from build123d import *

# Parameters (mm, degrees)
SKETCH1_R           = 1.5875
BOSS_EXTRUDE1_DEPTH = 6
CUT_EXTRUDE1_START  = 9
CUT_EXTRUDE1_DEPTH  = 2.1


with BuildPart() as part:
    # Sketch1 → Boss-Extrude1 (new body)
    with BuildSketch(Plane.XY):
        with BuildLine():
            Line((-9.16515139, -4), (-1.658312395, -2.5))
            ThreePointArc((-1.658312395, -2.5), (0, -3), (1.658312395, -2.5))
            Line((1.658312395, -2.5), (9.16515139, -4))
            ThreePointArc((9.16515139, -4), (10, 0), (9.16515139, 4))
            Line((9.16515139, 4), (1.658312395, 2.5))
            ThreePointArc((1.658312395, 2.5), (0, 3), (-1.658312395, 2.5))
            Line((-1.658312395, 2.5), (-9.16515139, 4))
            ThreePointArc((-9.16515139, 4), (-10, 0), (-9.16515139, -4))
        make_face()
        Circle(SKETCH1_R, mode=Mode.SUBTRACT)
    extrude(amount=BOSS_EXTRUDE1_DEPTH)

    # Sketch2 → Cut-Extrude1 (cut)
    with BuildSketch(Plane(origin=(0, 0, 0), x_dir=(0, 0, -1), z_dir=(1, 0, 0)).offset(CUT_EXTRUDE1_START)):
        with BuildLine():
            Line((-3, 2.1), (-5.1, 2.1))
            Line((-5.1, 2.1), (-5.1, -2.1))
            Line((-5.1, -2.1), (-3, -2.1))
            ThreePointArc((-3, -2.1), (-0.9, 0), (-3, 2.1))
        make_face()
    cut_extrude1 = extrude(amount=-CUT_EXTRUDE1_DEPTH, mode=Mode.SUBTRACT)

    # Mirror1: Cut-Extrude1 across plane
    add(cut_extrude1.mirror(Plane(origin=(0, 0, 0), x_dir=(0, 0, 1), z_dir=(1, 0, 0))), mode=Mode.SUBTRACT)


solid = part.part
The listing builds one solid part. Answer for the finished solid, in the listing's coordinates (mm). A direction names the side the tool comes from. Coordinates: 2 decimals unless noted, no trailing zeros. Order: outer loops, then holes, each group sorted by start corner. A loop starts at its lowest first (then second) coordinate and runs counter-clockwise, first axis right, second up. Notation, with made-up numbers: M 10.25,25 L 32.25,25 A10 cw 32.25,42 Z; hole C 14,-6.75 d5. An arc over 180 degrees is marked long. Use CSV: the item, a comma, the result in double quotes.
Q1. A tool of negligible diameter and unlimited length cuts with its end or side. For faces 4 (the flat face through (5.36, -3.24, 2.96)), 5 (the flat face through (0, -2, 0)), 6 (the flat face through (5.46, 3.26, 2.96)), 7 (the cylindrical face through (-0.34, -1.55, 2.96)), 8 (the flat face through (-6.9, 0, 3)), from which of +Z, -Z, +X, -X, +Y, -Y can it reach the whole face along a straight path? Write none if from no direction.
Here are the results:
face 4,"+Z, -Z, -Y"
face 5,"-Z, +X, -X, +Y, -Y"
face 6,"+Z, -Z, +Y"
face 7,"+Z, -Z"
face 8,"none"
Q2. Section B-B (z = 0.7) is taken. Determine the outline of the cut face in (x, y) (1 decimal).
Here are the results:
outline,"M -9.2,-4 L -1.7,-2.5 A3 ccw 1.7,-2.5 L 9.2,-4 A10 ccw 9.2,4 L 1.7,2.5 A3 ccw -1.7,2.5 L -9.2,4 A10 ccw Z; hole C 0,0 d3.2"
Q3. Section C-C (x = 0) is taken. Determine the outline of the cut face in (y, z).
Here are the results:
outline,"M -3,0 L -1.59,0 L -1.59,6 L -3,6 Z; M 1.59,0 L 3,0 L 3,6 L 1.59,6 Z"
Q4. Section A-A (y = 0) is taken. Determine the outline of the cut face in (x, z).
Here are the results:
outline,"M -10,0 L -1.59,0 L -1.59,6 L -10,6 Z; M 1.59,0 L 10,0 L 10,6 L 1.59,6 Z; hole M -9,0.9 L -6.9,0.9 L -6.9,5.1 L -9,5.1 Z; hole M 6.9,0.9 L 9,0.9 L 9,5.1 L 6.9,5.1 Z"
Q5. Straight lines are drawn through the part: L1, parallel to Y at x = 0, z = 2; L2, parallel to X at y = -0.75, z = 2.8; L3, parallel to Y at x = 0.5, z = 2.95. For each, find the intervals that lie inside material, in ascending order.
Here are the results:
L1,"-3 to -1.59, 1.59 to 3"
L2,"-9.97 to -9, -6.9 to -1.4, 1.4 to 6.9, 9 to 9.97"
L3,"-2.96 to -1.51, 1.51 to 2.96"
Q6. Determine the mould class of faces 1 (the cylindrical face through (-10, 0, 3)), 2 (the flat face through (-9, 0, 3)), 3 (the cylindrical face through (10, 0, 3)) for opening direction X: pulls with the +X half, pulls with the -X half, needs draft (parallel to the pull), parting line crosses it, or undercut.
Here are the results:
face 1,"pulls with the -X half"
face 2,"undercut"
face 3,"pulls with the +X half"
Q7. Given pin 1 Ø1 at (x, z) = (-2, 0.5) entering from -Y; pin 2 Ø3 at (x, y) = (-4, 1.5) entering from -Z; pin 3 Ø2 at (y, z) = (-1.5, 2.5) entering from +X; pin 4 Ø1.5 at (y, z) = (1.5, 1) entering from -X, each flat-ended and moving along its own axis, determine where each tip first touches the part or whether it passes through.
Here are the results:
pin 1,"y = -2.67"
pin 2,"z = 0"
pin 3,"x = 9.99"
pin 4,"x = -9.97"
Q8. Section D-D (y = 3.25) is taken. Determine the outline of the cut face in (x, z).
Here are the results:
outline,"M -9.46,0 L -5.41,0 L -5.41,6 L -9.46,6 Z; M 5.41,0 L 9.46,0 L 9.46,6 L 5.41,6 Z"
